Input: part model. Units: mm. Frame: model coordinates. Give positions to 0.01 mm unless a question says otherwise; leave off trailing zeros. Write each loop counter-clockwise with the first axis right and the second up, starting at its lowest first coordinate (ties: lowest second). Pieces come first, ordered by that corner, then holes. Notation, with made-up numbers: (-12.5, 41) - (-8.5, 41) arc R5 cw to (-8.5, 45) - close; hole circle Ø2 at (74, -1). An arc over 180 degrees is marked (long way). Answer as a JSON object with one key per item and string values. Group by question number.
from build123d import *

# Parameters (mm, degrees)
SKETCH1_W           = 40
SKETCH1_H           = 40
BOSS_EXTRUDE1_DEPTH = 20
SKETCH2_R           = 4.5
CUT_EXTRUDE1_DEPTH  = 49.989794856
SKETCH3_R           = 4.5
CUT_EXTRUDE2_DEPTH  = 49.989794856
FILLET1_R           = 1


with BuildPart() as part:
    # Sketch1 → Boss-Extrude1 (new, symmetric)
    with BuildSketch(Plane.XY):
        Rectangle(SKETCH1_W, SKETCH1_H)
    extrude(amount=BOSS_EXTRUDE1_DEPTH, both=True)

    # Sketch2 → Cut-Extrude1 (cut, through all)
    with BuildSketch(Plane.XY.offset(20)):
        with Locations((0, -9)):
            Circle(SKETCH2_R)
    extrude(amount=-CUT_EXTRUDE1_DEPTH, mode=Mode.SUBTRACT)

    # Sketch3 → Cut-Extrude2 (cut, through all)
    with BuildSketch(Plane.ZY.offset(20)):
        with Locations(Location((0, 9, 0), (0, 0, 270))):
            Circle(SKETCH3_R)
    extrude(amount=-CUT_EXTRUDE2_DEPTH, mode=Mode.SUBTRACT)

    # Fillet1
    fillet1_edges = [part.edges().sort_by_distance(p)[0] for p in [
        (-20, 0, 20),
        (-4.5, -9, -20),
        (-4.5, -9, 20),
        (0, -20, 20),
        (20, 13.5, 0),
        (-20, 13.5, 0),
        (20, 0, 20),
        (0, -20, -20),
        (-20, 0, -20),
        (0, 20, -20),
        (20, 0, -20),
        (20, -20, 0),
        (-20, -20, 0),
        (-20, 20, 0),
        (20, 20, 0),
        (0, 20, 20),
    ]]
    fillet(fillet1_edges, radius=FILLET1_R)


solid = part.part
1) Cut plane A-A on x = 0. Return the cut outline in (y, z).
2) Cut plane B-B on z = 0. Return the cut outline in (x, y).
3) Cut plane D-D on x = 17. Return the cut outline in (y, z).
4) Line query: line 1 along Y through (x, z) = (0, -7); line 2 along Y through (x, z) = (-4, 1); line 3 along X through (y, z) = (-10.5, 16.5). Output: solid intervals per line, ascending. Write a range as from..to.
5) Pin query (flat end, axial travel): P1, Ø10.5, axis at y = 9, z = 0, coming from the -X side. Return the tip coordinate at first contact, or that it passes through.
6) Mould query, pull axis X, two halves, no side actions, for faces 1 (the face through (-0.266, 4.708, 1.352)), 2 (the face through (-0.59, -4.54, 0.27)), 3 (the face through (20, 0, 0)). Classes: +X half, -X half, draft (parallel to the pull), parting line (faces both ways), or undercut.
7) Cut plane C-C on y = -9. Return the cut outline in (x, z), and give its area (3 significant figures).
Filled in:
{
 "1": {"outline": "(-20, -19) arc R1 ccw to (-19, -20) - (-14.5, -20) arc R1 ccw to (-13.5, -19) - (-13.5, 19) arc R1 ccw to (-14.5, 20) - (-19, 20) arc R1 ccw to (-20, 19) - close; (-4.5, -19) arc R1 ccw to (-3.5, -20) - (19, -20) arc R1 ccw to (20, -19) - (20, 19) arc R1 ccw to (19, 20) - (-3.5, 20) arc R1 ccw to (-4.5, 19) - close; hole circle Ø9 at (9, 0)"},
 "2": {"outline": "(-20, -19) arc R1 ccw to (-19, -20) - (19, -20) arc R1 ccw to (20, -19) - (20, 3.5) arc R1 ccw to (19, 4.5) - (-19, 4.5) arc R1 ccw to (-20, 3.5) - close; (-20, 14.5) arc R1 ccw to (-19, 13.5) - (19, 13.5) arc R1 ccw to (20, 14.5) - (20, 19) arc R1 ccw to (19, 20) - (-19, 20) arc R1 ccw to (-20, 19) - close; hole circle Ø9 at (0, -9)"},
 "3": {"outline": "(-20, -19) arc R1 ccw to (-19, -20) - (19, -20) arc R1 ccw to (20, -19) - (20, 19) arc R1 ccw to (19, 20) - (-19, 20) arc R1 ccw to (-20, 19) - close; hole circle Ø9 at (9, 0)"},
 "4": {"line 1": "y = -20..-13.5, -4.5..20", "line 2": "y = -20..-11.06, -6.94..4.61, 13.39..20", "line 3": "x = -20..-4.24, 4.24..20"},
 "5": {"P1": "stops at x = -19.97"},
 "6": {"face 1": "draft", "face 2": "undercut", "face 3": "+X half"},
 "7": {"outline": "(-20, -19) arc R1 ccw to (-19, -20) - (-5.5, -20) arc R1 ccw to (-4.5, -19) - (-4.5, 19) arc R1 ccw to (-5.5, 20) - (-19, 20) arc R1 ccw to (-20, 19) - close; (4.5, -19) arc R1 ccw to (5.5, -20) - (19, -20) arc R1 ccw to (20, -19) - (20, 19) arc R1 ccw to (19, 20) - (5.5, 20) arc R1 ccw to (4.5, 19) - close", "area": "1,240 mm²"}
}
